```python
from build123d import *

# Parameters (mm, degrees)
SKETCH_1_W             = 135
SKETCH_1_H             = 40
SKETCH_1_R             = 3.5
SM_BASE_FLANGE_1_DEPTH = 1
CHAMFER_1_SIZE         = 15


# Sheet-metal steps are written as plain solids
with BuildPart() as part:
    # Sketch 1 → Базовая кромка1 (new body)
    with BuildSketch(Plane.XY):
        Rectangle(SKETCH_1_W, SKETCH_1_H)
        with Locations((-57.5, 0)):
            Circle(SKETCH_1_R, mode=Mode.SUBTRACT)
        with Locations(Location((57.5, 0, 0), (0, 0, 180))):
            Circle(SKETCH_1_R, mode=Mode.SUBTRACT)
    extrude(amount=-SM_BASE_FLANGE_1_DEPTH)

    # Фаска1
    chamfer_1_edges = [part.edges().sort_by_distance(p)[0] for p in [
        (-67.5, -20, -0.5),
    ]]
    chamfer(chamfer_1_edges, length=CHAMFER_1_SIZE)


solid = part.part
```
Read the model definition and answer for the solid it produces. Units are mm, in the model's axes. Give positions to 0.01 mm unless a question says otherwise; leave off trailing zeros. Write each loop counter-clockwise with the first axis right and the second up, starting at its lowest first coordinate (ties: lowest second). Pieces come first, ordered by that corner, then holes. Notation, with made-up numbers: (-34, -11) -> (23, -11) arc R28 ccw to (23, 28) -> close; hole circle Ø3 at (81, 51.5). An arc over 180 degrees is marked (long way). Answer in a Markdown table with one row per item.
1) Section D-D on x = -57.5 is taken. Give the vertices of the cut face in (y, z), plus the area to 3 significant figures.
Results list:
| item | result |
|---|---|
| outline | (-15, -1) -> (-3.5, -1) -> (-3.5, 0) -> (-15, 0) -> close; (3.5, -1) -> (20, -1) -> (20, 0) -> (3.5, 0) -> close |
| area | 28.0 mm^2 |
2) Section B-B on y = 0 is taken. Give the vertices of the cut face in (x, z), plus the area to 3 significant figures.
Results list:
| item | result |
|---|---|
| outline | (-67.5, -1) -> (-61, -1) -> (-61, 0) -> (-67.5, 0) -> close; (-54, -1) -> (54, -1) -> (54, 0) -> (-54, 0) -> close; (61, -1) -> (67.5, -1) -> (67.5, 0) -> (61, 0) -> close |
| area | 121 mm^2 |
3) Section A-A on x = 57.5 is taken. Give the vertices of the cut face in (y, z), plus the area to 3 significant figures.
Results list:
| item | result |
|---|---|
| outline | (-20, -1) -> (-3.5, -1) -> (-3.5, 0) -> (-20, 0) -> close; (3.5, -1) -> (20, -1) -> (20, 0) -> (3.5, 0) -> close |
| area | 33.0 mm^2 |
4) Section C-C on z = -0.75 is taken. Give the vertices of the cut face in (x, y), plus the area to 3 significant figures.
Results list:
| item | result |
|---|---|
| outline | (-67.5, -5) -> (-52.5, -20) -> (67.5, -20) -> (67.5, 20) -> (-67.5, 20) -> close; hole circle Ø7 at (-57.5, 0); hole circle Ø7 at (57.5, 0) |
| area | 5,210 mm^2 |
5) Straight lines are drawn through the part: line 1 (X direction, y = -2.5, z = -0.7); line 2 (Y direction, x = 57.5, z = -0.3); line 3 (X direction, y = -11.5, z = -0.95). For each, find the intervals that lie inside material, in ascending order. Write a range as [from, to].
Results list:
| item | result |
|---|---|
| line 1 | [-67.5, -59.95], [-55.05, 55.05], [59.95, 67.5] |
| line 2 | [-20, -3.5], [3.5, 20] |
| line 3 | [-61, 67.5] |
6) Determine the mould class of faces 1 (the flat face through (-1, 0, -1)), 2 (the flat face through (-59.9, -12.6, -0.5)), 3 (the cylindrical face through (-60.997, 0.154, -0.493)) for opening direction X: released by +X, released by -X, zero draft, split by the parting line, or undercut.
Results list:
| item | result |
|---|---|
| face 1 | zero draft |
| face 2 | released by -X |
| face 3 | undercut |
